from build123d import *

# Parameters (mm, degrees)
SKETCH8_W           = 57.15
SKETCH8_H           = 127
BOSS_EXTRUDE3_DEPTH = 5.334
SKETCH9_R           = 16.505180298
CUT_EXTRUDE4_DEPTH  = 140.368483008
SKETCH12_W          = 19.05
SKETCH12_H          = 5.334
CUT_EXTRUDE8_DEPTH  = 5.334
SKETCH14_W          = 10.414
SKETCH14_H          = 5.334
BOSS_EXTRUDE4_DEPTH = 5.334
SKETCH15_W          = 5.207
SKETCH15_H          = 5.334
CUT_EXTRUDE9_DEPTH  = 5.334
SKETCH22_W          = 19.05
SKETCH22_H          = 5.334
BOSS_EXTRUDE5_DEPTH = 10.668
SKETCH23_W          = 8.89
SKETCH23_H          = 5.334
CUT_EXTRUDE15_DEPTH = 145.245837417
SKETCH24_W          = 5.334
SKETCH24_H          = 5.08
CUT_EXTRUDE16_DEPTH = 145.245837417


with BuildPart() as part:
    # Sketch8 → Boss-Extrude3 (new body)
    with BuildSketch(Plane.XY):
        with Locations((28.575, 63.5)):
            Rectangle(SKETCH8_W, SKETCH8_H)
    extrude(amount=BOSS_EXTRUDE3_DEPTH)

    # Sketch9 → Cut-Extrude4 (cut, through all)
    with BuildSketch(Plane.XY.offset(5.334)):
        with BuildLine():
            Line((46.736, 127), (10.414, 127))
            Line((10.414, 127), (12.069819702, 29.083))
            ThreePointArc((12.069819702, 29.083), (28.575, 45.588180298), (45.080180298, 29.083))
            Line((45.080180298, 29.083), (46.736, 127))
        make_face()
        with Locations((28.575, 29.083)):
            Circle(SKETCH9_R)
    extrude(amount=-CUT_EXTRUDE4_DEPTH, mode=Mode.SUBTRACT)

    # Sketch12 → Cut-Extrude8 (cut)
    with BuildSketch(Plane(origin=(0, 0, 0), x_dir=(-1, 0, 0), z_dir=(0, -1, 0))):
        with Locations((-47.625, -2.667)):
            Rectangle(SKETCH12_W, SKETCH12_H)
        with Locations((-9.525, -2.667)):
            Rectangle(SKETCH12_W, SKETCH12_H)
    extrude(amount=-CUT_EXTRUDE8_DEPTH, mode=Mode.SUBTRACT)

    # Sketch14 → Boss-Extrude4 (add)
    with BuildSketch(Plane(origin=(0, 127, 0), x_dir=(1, 0, 0), z_dir=(0, 1, 0))):
        with Locations((51.943, -2.667)):
            Rectangle(SKETCH14_W, SKETCH14_H)
        with Locations((5.207, -2.667)):
            Rectangle(SKETCH14_W, SKETCH14_H)
    extrude(amount=BOSS_EXTRUDE4_DEPTH)

    # Sketch15 → Cut-Extrude9 (cut)
    with BuildSketch(Plane(origin=(0, 132.334, 0), x_dir=(1, 0, 0), z_dir=(0, 1, 0))):
        with Locations((7.8105, -2.667)):
            Rectangle(SKETCH15_W, SKETCH15_H)
        with Locations((49.3395, -2.667)):
            Rectangle(SKETCH15_W, SKETCH15_H)
    extrude(amount=-CUT_EXTRUDE9_DEPTH, mode=Mode.SUBTRACT)

    # Sketch22 → Boss-Extrude5 (add)
    with BuildSketch(Plane.XZ):
        with Locations((28.575, 2.667)):
            Rectangle(SKETCH22_W, SKETCH22_H)
    extrude(amount=BOSS_EXTRUDE5_DEPTH)

    # Sketch23 → Cut-Extrude15 (cut, through all)
    with BuildSketch(Plane(origin=(0, 0, 0), x_dir=(-1, 0, 0), z_dir=(0, 0, -1))):
        with Locations((-28.575, -2.667)):
            Rectangle(SKETCH23_W, SKETCH23_H)
    extrude(amount=-CUT_EXTRUDE15_DEPTH, mode=Mode.SUBTRACT)

    # Sketch24 → Cut-Extrude16 (cut, through all)
    with BuildSketch(Plane(origin=(0, 0, 0), x_dir=(-1, 0, 0), z_dir=(0, 0, -1))):
        with Locations((-54.483, 12.954)):
            Rectangle(SKETCH24_W, SKETCH24_H)
        with Locations((-2.667, 12.954)):
            Rectangle(SKETCH24_W, SKETCH24_H)
    extrude(amount=-CUT_EXTRUDE16_DEPTH, mode=Mode.SUBTRACT)


solid = part.part
The model under review builds one solid part; all positions refer to its coordinate system, in mm. A direction names the side the tool comes from. Round coordinates to 2 decimals unless told otherwise and drop trailing zeros. Loops run counter-clockwise (first coordinate to the right, second up) from the corner with the lowest first, then second, coordinate; pieces in that order, holes last. Notation, with made-up numbers: M -16,22.25 L 39,22.25 A18 ccw 39,36.25 Z; hole C 19.25,3 d8. An arc over 180 degrees is marked long. Answer as a JSON object with one key per item and string values.
Item 1: We need section A-A, the plane y = 39.5. State the section outline as (x, z) points.
Check sheet entries:
{"outline": "M 0,0 L 11.89,0 L 11.89,5.33 L 0,5.33 Z; M 45.26,0 L 57.15,0 L 57.15,5.33 L 45.26,5.33 Z"}
Item 2: We need section D-D, the plane x = 22. State the section outline as (y, z) points.
Check sheet entries:
{"outline": "M -10.67,0 L 13.94,0 L 13.94,5.33 L -10.67,5.33 Z"}
Item 3: For line 1 along Y through (x, z) = (2, 2.55); line 2 along X through (y, z) = (2, 5.05); line 3 along X through (y, z) = (22, 3.05), list the stretches that pass through material, from the lowest coordinate up.
Check sheet entries:
{"line 1": "5.33 to 10.41, 15.49 to 132.33", "line 2": "19.05 to 38.1", "line 3": "0 to 13.67, 43.48 to 57.15"}
Item 4: Clearance check with flat-ended pins moving along their axes: P1, Ø1.6, axis at y = -2.5, z = 1.5, coming from the -X side; P2, Ø1.6, axis at y = -4.5, z = 2.5, coming from the -X side; P3, Ø1.6, axis at x = 2.5, z = 2.5, coming from the -Y side; P4, Ø3, axis at y = 111.5, z = 3.5, coming from the -X side. State where each tip first meets the part, or that it passes through.
Check sheet entries:
{"P1": "x = 19.05", "P2": "x = 19.05", "P3": "y = 5.33", "P4": "x = 0"}
Item 5: Tool access review of faces 1 (the face through (33.02, -3, 3)), 2 (the face through (5.334, 13, 3)), 3 (the face through (55, 10.414, 3)): name each direction out of +Z, -Z, +X, -X, +Y, -Y from which nothing blocks a thin tool from reaching the whole face with its end or side.
Check sheet entries:
{"face 1": "+Z, -Z", "face 2": "+Z, -Z, -X", "face 3": "+Z, -Z, +X"}
Item 6: We need section C-C, the plane y = 80. State the section outline as (x, z) points.
Check sheet entries:
{"outline": "M 0,0 L 11.21,0 L 11.21,5.33 L 0,5.33 Z; M 45.94,0 L 57.15,0 L 57.15,5.33 L 45.94,5.33 Z"}
Item 7: We need section B-B, the plane z = 3.8. State the section outline as (x, y) points (3 decimals).
Check sheet entries:
{"outline": "M 0,5.334 L 19.05,5.334 L 19.05,-10.668 L 38.1,-10.668 L 38.1,5.334 L 57.15,5.334 L 57.15,10.414 L 51.816,10.414 L 51.816,15.494 L 57.15,15.494 L 57.15,132.334 L 51.943,132.334 L 51.943,127 L 46.736,127 L 45.08,29.083 A16.505 cw 12.07,29.083 L 10.414,127 L 5.207,127 L 5.207,132.334 L 0,132.334 L 0,15.494 L 5.334,15.494 L 5.334,10.414 L 0,10.414 Z; hole M 24.13,-5.334 L 33.02,-5.334 L 33.02,0 L 24.13,0 Z"}
Item 8: The part is to be moulded in two halves that separate along Y. For faces 4 (the face through (51.816, 13, 3)), 5 (the face through (19.05, -3, 3)), 6 (the face through (49, 127, 3)), say which applies: +Y half, -Y half, draft (parallel to the pull), parting line (faces both ways), or undercut.
Check sheet entries:
{"face 4": "undercut", "face 5": "draft", "face 6": "+Y half"}
